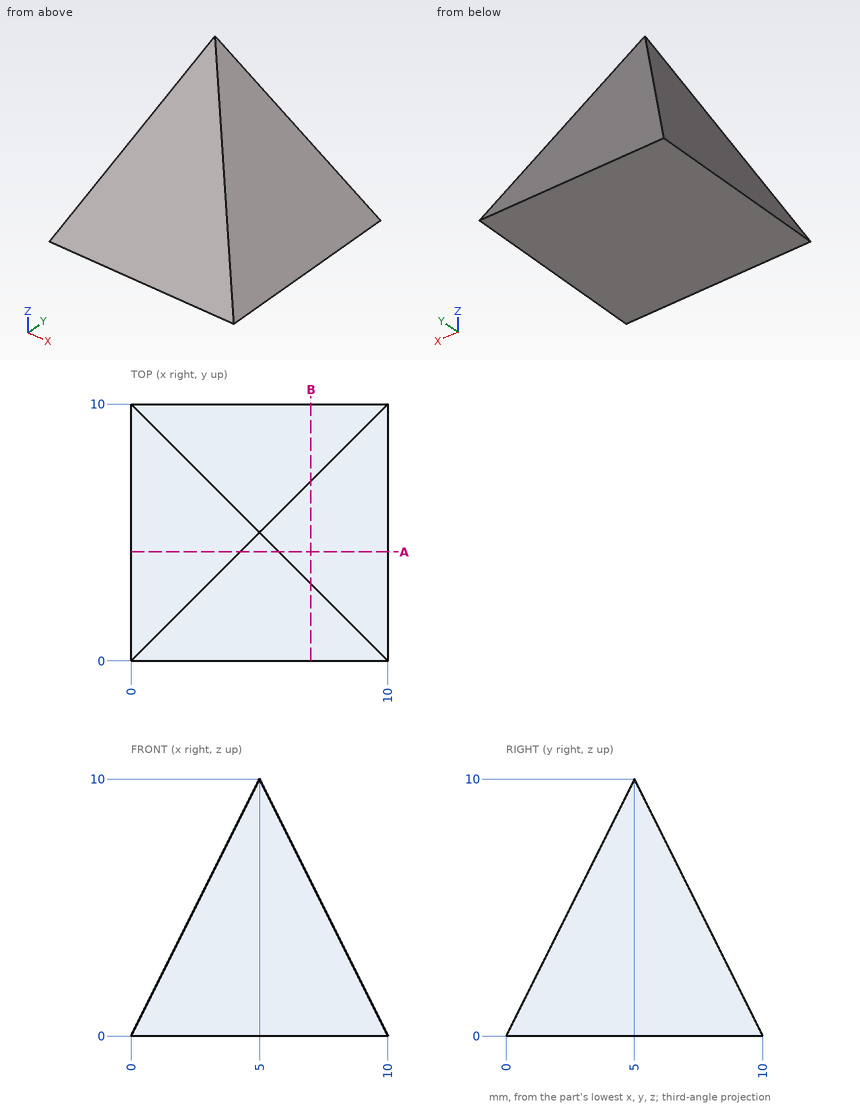
Geometry: see drawing. Coordinates: mm, zero at the bounding-box minimum. Give positions to 0.01 mm unless a question says otherwise; leave off trailing zeros. Loops run counter-clockwise (first coordinate to the right, second up) from the corner with the lowest first, then second, coordinate; pieces in that order, holes last. Notation, with made-up numbers: (11, -30) -> (25, -30) arc R22 cw to (25, 5) -> close; hole circle Ø3 at (13.5, 18.25). An arc over 180 degrees is marked (long way). Put each result on its own line as item: value.
1. Cut plane B-B (x = 7). Return the cut outline in (y, z), plus the area to 3 significant figures.
Taken from the geometry:
outline: (0, 0) -> (10, 0) -> (7, 6) -> (3, 6) -> close
area: 42.0 mm2
2. Ray query, line 1 along X through (y, z) = (5.75, 3.25) (3 decimals); line 2 along Z through (x, y) = (1.5, 5.75); line 3 along X through (y, z) = (5.25, 0.5). Return the intervals inside material, ascending. Write a range as [from, to].
Taken from the geometry:
line 1: x = [1.625, 8.375]
line 2: z = [0, 3]
line 3: x = [0.25, 9.75]
3. Cut plane A-A (y = 4.25). Return the cut outline in (x, z).
Taken from the geometry:
outline: (0, 0) -> (10, 0) -> (5.75, 8.5) -> (4.25, 8.5) -> close
4. Pin query (flat end, axial travel): P1, Ø1, axis at y = 5.5, z = 8.5, coming from the -X side; P2, Ø3, axis at x = 7.5, y = 7.5, coming from the +Z side; P3, Ø1.5, axis at x = 5.5, z = 9, coming from the +Y side (3 decimals). Return the tip coordinate at first contact, or that it passes through.
Taken from the geometry:
P1: stops at x = 4
P2: stops at z = 7.12
P3: stops at y = 5.875
